Autodesk Inventor part; units mm, degrees
ref_plane "YZ Plane" through (0, 0, 0) normal (1, 0, 0) x (0, 1, 0)
ref_plane "XZ Plane" through (0, 0, 0) normal (0, 1, 0) x (-1, 0, 0)
ref_plane "XY Plane" through (0, 0, 0) normal (0, 0, 1) x (1, 0, 0)
sketch "Esboço1" plane through (0, 0, 0) normal (0, 0, 1) x (1, 0, 0)
  circle A0 centre (9.5, -2.575) radius 10.5 construction
  line L0 (21.9348, 5.0533) -> (21.9348, -29.9467) construction
  line L1 (-3.0652, -29.9467) -> (-3.0652, 5.0533) construction
  circle A1 centre (9.5, -2.575) radius 10.575 construction
  line L2 (21.9348, -13.15) -> (-3.0652, -13.15) construction
  line L3 (9.4348, -13.15) -> (9.4348, 4.425) construction
  line L4 (-5.5652, 24.425) -> (24.4348, 24.425)
  line L5 (24.4348, 24.425) -> (24.4348, -15.575)
  line L6 (24.4348, -15.575) -> (-5.5652, -15.575)
  line L7 (-5.5652, -15.575) -> (-5.5652, 24.425)
  line L8 (-5.5652, 24.425) -> (24.4348, -15.575) construction
  line L9 (24.4348, 24.425) -> (-5.5652, -15.575) construction
  point P0 (0, 0)
  dimension "d1" = 21.15
  dimension "d3" = 30
  dimension "d4" = 40
  dimension "d51" = 13
extrude "Extrusão1" add sketch "Esboço1" against normal blind 50
sketch "Esboço2" plane through (0, 0, 0) normal (0, 0, 1) x (1, 0, 0)
  circle A0 centre (9.4348, -2.575) radius 5.995 construction
  line L0 (24.4348, -15.575) -> (-5.5652, -15.575)
  line L1 (-5.5652, -15.575) -> (-5.5652, 24.425)
  dimension "d52" = 13
  dimension "d53" = 15
hole "Furo1" at (9.4348, -2.575, 0) direction (0, 0, -1) diameter 13 end through all counterbore diameter 21.2 counterbore depth 32
sketch "Esboço3" plane through (-5.5652, -15.575, 0) normal (-1, 0, 0) x (0, 0, 1)
  line L0 (-50, 0) -> (-50, 40) construction
  line L1 (0, 40) -> (0, 0) construction
  line L2 (-50, 40) -> (0, 40) construction
  line L3 (0, 40) -> (0, 0) construction
  line L4 (0, 0) -> (-50, 0) construction
  line L5 (-50, 0) -> (-50, 40) construction
  line L6 (0, 15.575) -> (-50, 15.575) construction
  line L7 (-35, 15.575) -> (-35, 40) construction
hole "Furo2" at (-5.5652, 0, -35) direction (1, 0, 0) diameter 4.917 depth 13 tip angle 118
sketch "Esboço4" plane through (-5.5652, -15.575, 0) normal (-1, 0, 0) x (0, 0, 1)
  line L0 (-50, 30.5) -> (-20, 30.5)
  line L1 (-20, 30.5) -> (-20, 40)
  line L2 (-20, 40) -> (-50, 40)
  line L3 (-50, 40) -> (-50, 30.5)
  point P0 (0, 15.575)
  point P1 (-50, 0)
  dimension "d22" = 30.5
  dimension "d23" = 30
extrude "Extrusão2" cut sketch "Esboço4" against normal blind 31.25
sketch "Esboço6" plane through (24.4348, -15.575, 0) normal (1, 0, 0) x (0, 0, -1)
  circle A0 centre (35, 15.575) radius 2.4585 construction
  circle A1 centre (35, 15.575) radius 2.4585 construction
  point P0 (0, 15.575)
hole "Furo3" at (24.4348, 0, -35) direction (-1, 0, 0) diameter 4.917 depth 13 tip angle 118
sketch "Esboço7" plane through (-5.5652, -15.575, 0) normal (0, -1, 0) x (1, 0, 0)
  line L0 (0, 0) -> (30, 0)
  line L1 (15, 0) -> (15, -16) construction
  point P0 (5.5652, 0)
  dimension "d33" = 16
hole "Furo4" at (9.4348, -15.575, -16) direction (0, 1, 0) diameter 3.242 depth 5.18 tip angle 118
sketch "Esboço8" plane through (-5.5652, 14.925, -20) normal (0, 1, 0) x (1, 0, 0)
  line L0 (30, 0) -> (0, 0)
  line L1 (30, 30) -> (0, 30)
  line L2 (30, -20) -> (30, 30)
  line L3 (0, -20) -> (0, 30)
  line L4 (15, 0) -> (15, 7.5) construction
  line L5 (15, 30) -> (15, 22.5) construction
  point P0 (5.5652, -20)
  dimension "d41" = 7.5
  dimension "d42" = 7.5
hole "Furo5" at (9.4348, 14.925, -27.5) at (9.4348, 14.925, -42.5) direction (0, -1, 0) diameter 3.242 depth 5.5 tip angle 118
properties part number "carro_do_rolamento_direito" material "Alumínio 6061"
Geometry: final body of the model. Coordinates: model frame, mm. A direction names the side the tool comes from. Round coordinates to 2 decimals unless told otherwise and drop trailing zeros. Loops run counter-clockwise (first coordinate to the right, second up) from the corner with the lowest first, then second, coordinate; pieces in that order, holes last.
Q1. Section B-B on y = -6.5. Return loops of the section in (x, z), plus the area to 3 significant figures.
Q2. Section C-C on x = 6. Return loops of the section in (y, z) (3 decimals).
Q3. Pull-direction query (Z, two-part tool) for faces 5 (the cylindrical face through (8.339, 12.137, -43.695)), 6 (the flat face through (14, 2.3, -32)), 7 (the flat face through (10, -15.575, -25)); classes: released by +Z, released by -Z, zero draft, split by the parting line, or undercut.
Q4. Pin query (flat end, axial travel): P1, Ø8, axis at x = 9.43, y = -2.58, coming from the -Z side; P2, Ø8, axis at y = 0, z = -35, coming from the -X side; P3, Ø17, axis at x = 9.43, y = -2.58, coming from the +Z side; P4, Ø3, axis at x = 9.43, z = -42.5, coming from the +Y side. Return the tip coordinate at first contact, or that it passes through.
Q5. Access query for faces 1 (the cylindrical face through (-1.075, -1.195, -16.224)), 2 (the cylindrical face through (9.36, 12.14, -29.12)), 3 (the cylindrical face through (8.948, -14.295, -17.546)), 4 (the flat face through (9, 20, -20)). Directions: +Z, -Z, +X, -X, +Y, -Y. A direction counts if a zero-diameter tool reaches every point of the face in a straight line with its end or side. Return the directions, or none.
Q6. Section D-D on x = 0.5. Return loops of the section in (y, z) (1 decimal), plus the area to 3 significant figures.
Q7. Material intervals for L1, parallel to Y at x = 20, z = -35 (1 decimal); L2, parallel to X at y = -3, z = -21.5; L3, parallel to Y at x = 9, z = -36 (3 decimals), sorted ascending.
Q8. Section A-A on z = -35. Return loops of the section in (x, y) (1 decimal), plus the area to 3 significant figures.
Evaluation:
1. outline: (-5.57, -50) - (4.25, -50) - (4.25, -32) - (-0.41, -32) - (-0.41, 0) - (-5.57, 0) - close; (14.62, -50) - (24.43, -50) - (24.43, 0) - (19.28, 0) - (19.28, -32) - (14.62, -32) - close
1. area: 683 mm2
2. outline: (-15.575, -50) - (-8.093, -50) - (-8.093, -32) - (-12.603, -32) - (-12.603, 0) - (-15.575, 0) - close; (2.943, -50) - (14.925, -50) - (14.925, -20) - (24.425, -20) - (24.425, 0) - (7.453, 0) - (7.453, -32) - (2.943, -32) - close
3. face 5: undercut
3. face 6: released by +Z
3. face 7: zero draft
4. P1: passes through
4. P2: stops at x = -5.57
4. P3: stops at z = -32
4. P4: stops at y = 9.36
5. face 1: +Z
5. face 2: +Y
5. face 3: -Y
5. face 4: -Z, +X, -X, +Y
6. outline: (-15.6, -50) - (14.9, -50) - (14.9, -20) - (24.4, -20) - (24.4, 0) - (3.1, 0) - (3.1, -32) - (-8.3, -32) - (-8.3, 0) - (-15.6, 0) - close; hole circle Ø4.9 at (0, -35)
6. area: 1,330 mm2
7. L1: y = -15.6 to -2.5, 2.5 to 14.9
7. L2: x = -5.57 to -1.16, 20.03 to 24.43
7. L3: y = -15.575 to -9.06, 3.91 to 14.925
8. outline: (-5.6, -15.6) - (24.4, -15.6) - (24.4, -2.5) - (15.9, -2.5) arc R6.5 cw (long way) to (2.9, -2.5) - (-5.6, -2.5) - close; (-5.6, 2.5) - (5.3, 2.5) arc R6.5 cw to (13.5, 2.5) - (24.4, 2.5) - (24.4, 14.9) - (-5.6, 14.9) - close
8. area: 691 mm2
